Geometry: final body of the model. Coordinates: model frame, mm. A direction names the side the tool comes from. Give positions to 0.01 mm unless a question says otherwise; leave off trailing zeros. Write each loop counter-clockwise with the first axis right and the second up, starting at its lowest first coordinate (ties: lowest second). Pieces come first, ordered by that corner, then holes. Notation, with made-up numbers: M -6,27.25 L 36,27.25 A17 cw 36,49.25 Z; hole C 88.5,-13.75 d11. An arc over 180 degrees is marked long. Use a Markdown table: item, result. Add a question column.
1) Section A-A on z = -14. Return the cut outline in (x, y), then the cut area to 3 significant figures.
2) Section C-C on y = 0.15. Return the cut outline in (x, z).
3) Section B-B on x = -23.5. Return the cut outline in (y, z), then the cut area to 3 significant figures.
4) Line query: line 1 (Z direction, x = -20.5, y = 0.4); line 2 (Y direction, x = -12, z = -2.5); line 3 (Z direction, x = -20, y = 0.9). Output: solid intervals per line, ascending.
5) Draft query along Y for faces 1 (the flat face through (-25, -1.25, 0)), 2 (the flat face through (-25, 0, -20)), 3 (the flat face through (-25, 0, -20.562)), 4 (the flat face through (-25, -1, 0)). Return one class per face: +Y half, -Y half, draft (parallel to the pull), parting line (faces both ways), or undercut.
6) Set-up query: faces 5 (the flat face through (-25, 0, 20.438)), 6 (the flat face through (-25, 0, 20)). Return all of +Z, -Z, +X, -X, +Y, -Y with unobstructed straight access to the full face (end or side cutting, diameter ignored); none if empty.
```python
from build123d import *

# Parameters (mm, degrees)
F2_DEPTH = 50
F3_DEPTH = 50.001


with BuildPart() as f2:
    # F1 (on Right) → F2 (new body)
    with BuildSketch(Plane.YZ):
        with BuildLine():
            ThreePointArc((0.75, -20.561926), (1.103553, -20.415479), (1.25, -20.061926))
            Line((1.25, -20.061926), (1.25, 19.938074))
            ThreePointArc((1.25, 19.938074), (1.103553, 20.291627), (0.75, 20.438074))
            Line((0.75, 20.438074), (-0.75, 20.438074))
            ThreePointArc((-0.75, 20.438074), (-1.103553, 20.291627), (-1.25, 19.938074))
            Line((-1.25, 19.938074), (-1.25, -20.061926))
            ThreePointArc((-1.25, -20.061926), (-1.103553, -20.415479), (-0.75, -20.561926))
            Line((-0.75, -20.561926), (0.75, -20.561926))
        make_face()
    extrude(amount=-F2_DEPTH)

    # F0 (on Right) → F3 (cut, through all)
    with BuildSketch(Plane.YZ):
        Polygon((1, -20), (1, 0), (1, 20), (-1, 20), (-1, -20), align=None)
    extrude(amount=-F3_DEPTH, mode=Mode.SUBTRACT)


solid = f2.part
```
Found:
| question | item | result |
|---|---|---|
| 1 | outline | M -50,-1.25 L 0,-1.25 L 0,-1 L -50,-1 Z; M -50,1 L 0,1 L 0,1.25 L -50,1.25 Z |
| 1 | area | 25.0 mm² |
| 2 | outline | M -50,-20.56 L 0,-20.56 L 0,-20 L -50,-20 Z; M -50,20 L 0,20 L 0,20.44 L -50,20.44 Z |
| 3 | outline | M -1.25,-20.06 A0.5 ccw -0.75,-20.56 L 0.75,-20.56 A0.5 ccw 1.25,-20.06 L 1.25,19.94 A0.5 ccw 0.75,20.44 L -0.75,20.44 A0.5 ccw -1.25,19.94 Z; hole M -1,-20 L 1,-20 L 1,20 L -1,20 Z |
| 3 | area | 22.3 mm² |
| 4 | line 1 | -20.56 to -20, 20 to 20.44 |
| 4 | line 2 | -1.25 to -1, 1 to 1.25 |
| 4 | line 3 | -20.54 to -20, 20 to 20.42 |
| 5 | face 1 | -Y half |
| 5 | face 2 | undercut |
| 5 | face 3 | draft |
| 5 | face 4 | undercut |
| 6 | face 5 | +Z, +X, -X, +Y, -Y |
| 6 | face 6 | +X, -X |
